```python
from build123d import *

# Parameters (mm, degrees)
F0_W     = 58
F0_H     = 36
F0_R     = 1.25
F0_R_2   = 1.2
F1_DEPTH = 9
F0_R_3   = 1
F2_DEPTH = 5.5
F3_DEPTH = 9
F4_R     = 3
F5_SIZE  = 2
F6_DEPTH = 10


with BuildPart() as f1:
    # F0 (on Top) → F1 (new body)
    with BuildSketch(Plane.XY):
        with Locations((22.1260370687, 12.181818096)):
            Rectangle(F0_W, F0_H)
        with Locations((-2.8739629313, -1.818181904)):
            Circle(F0_R, mode=Mode.SUBTRACT)
        with Locations((3.1260370687, -2.818181904)):
            Circle(F0_R_2, mode=Mode.SUBTRACT)
        with Locations((41.1260370687, -2.818181904)):
            Circle(F0_R_2, mode=Mode.SUBTRACT)
        with Locations((47.1260370687, -1.818181904)):
            Circle(F0_R, mode=Mode.SUBTRACT)
        with BuildLine():
            Line((-0.0042433119, 0.0237876128), (-0.0123524841, 0.02397218))
            Line((-0.0123524841, 0.02397218), (-0.0123524841, 0.0693824727))
            ThreePointArc((-0.0123524841, 0.0693824727), (-1.0671188126, 12.0466773263), (-0.0123524841, 24.02397218))
            ThreePointArc((-0.0123524841, 24.02397218), (22.4498159336, 26.0118318189), (44.9770614896, 25))
            ThreePointArc((44.9770614896, 25), (46.474513746, 12), (44.9770614896, -1))
            ThreePointArc((44.9770614896, -1), (22.4574664967, -1.8971785964), (0, 0))
            ThreePointArc((0, 0), (-0.0021227043, 0.0118936194), (-0.0042433119, 0.0237876128))
        make_face(mode=Mode.SUBTRACT)
        with Locations((-2.8739629313, 26.181818096)):
            Circle(F0_R, mode=Mode.SUBTRACT)
        with Locations((3.1260370687, 27.381818096)):
            Circle(F0_R_2, mode=Mode.SUBTRACT)
        with Locations((41.1260370687, 27.381818096)):
            Circle(F0_R_2, mode=Mode.SUBTRACT)
        with Locations((47.1260370687, 26.181818096)):
            Circle(F0_R, mode=Mode.SUBTRACT)
    extrude(amount=F1_DEPTH)

    # F0 (on Top) → F2 (join)
    with BuildSketch(Plane.XY):
        with BuildLine():
            Line((-0.0123524841, 24.02397218), (-0.0123524841, 0.0693824727))
            ThreePointArc((-0.0123524841, 0.0693824727), (-0.0083017494, 0.0465843578), (-0.0042433119, 0.0237876128))
            Line((-0.0042433119, 0.0237876128), (44.9770614896, -1))
            Line((44.9770614896, -1), (44.9770614896, 25))
            Line((44.9770614896, 25), (-0.0123524841, 24.02397218))
        make_face()
        with Locations((2.9444331303, 2.0848012064)):
            Circle(F0_R_3, mode=Mode.SUBTRACT)
        with Locations((41.6948273778, 2.0848012064)):
            Circle(F0_R_3, mode=Mode.SUBTRACT)
        with Locations((18.8074270263, 12.2937392443)):
            Circle(F0_R_3, mode=Mode.SUBTRACT)
        with Locations((2.9444331303, 21.6664075851)):
            Circle(F0_R_3, mode=Mode.SUBTRACT)
        with Locations((26.8074270263, 12.2937392443)):
            Circle(F0_R_3, mode=Mode.SUBTRACT)
        with Locations((41.6948273778, 21.6664075851)):
            Circle(F0_R_3, mode=Mode.SUBTRACT)
        with Locations((2.9444331303, 21.6664075851)):
            Circle(F0_R_3)
        with Locations((2.9444331303, 2.0848012064)):
            Circle(F0_R_3)
        with Locations((41.6948273778, 2.0848012064)):
            Circle(F0_R_3)
        with Locations((41.6948273778, 21.6664075851)):
            Circle(F0_R_3)
        with BuildLine():
            ThreePointArc((44.9770614896, 25), (22.4498159336, 26.0118318189), (-0.0123524841, 24.02397218))
            Line((-0.0123524841, 24.02397218), (44.9770614896, 25))
        make_face()
        with BuildLine():
            Line((44.9770614896, -1), (-0.0042433119, 0.0237876128))
            ThreePointArc((-0.0042433119, 0.0237876128), (-0.0021227043, 0.0118936194), (0, 0))
            ThreePointArc((0, 0), (22.4574664967, -1.8971785964), (44.9770614896, -1))
        make_face()
        with BuildLine():
            Line((44.9770614896, 25), (44.9770614896, -1))
            ThreePointArc((44.9770614896, -1), (46.474513746, 12), (44.9770614896, 25))
        make_face()
        with BuildLine():
            ThreePointArc((-0.0123524841, 24.02397218), (-1.0671188126, 12.0466773263), (-0.0123524841, 0.0693824727))
            Line((-0.0123524841, 0.0693824727), (-0.0123524841, 24.02397218))
        make_face()
    extrude(amount=F2_DEPTH)

    # F0 (on Top) → F3 (join)
    with BuildSketch(Plane.XY):
        with Locations((41.6948273778, 21.6664075851)):
            Circle(F0_R_3)
        with Locations((2.9444331303, 21.6664075851)):
            Circle(F0_R_3)
        with Locations((2.9444331303, 2.0848012064)):
            Circle(F0_R_3)
        with Locations((41.6948273778, 2.0848012064)):
            Circle(F0_R_3)
    extrude(amount=F3_DEPTH)

    # F4
    f4_edges = [f1.edges().sort_by_distance(p)[0] for p in [
        (51.126037, 30.181818, 4.5),
        (51.126037, -5.818182, 4.5),
        (-6.873963, -5.818182, 4.5),
        (-6.873963, 30.181818, 4.5),
    ]]
    fillet(f4_edges, radius=F4_R)

    # F5
    f5_edges = [f1.edges().sort_by_distance(p)[0] for p in [
        (-4.123963, -1.818182, 0),
        (-4.123963, 26.181818, 0),
        (45.876037, -1.818182, 0),
        (45.876037, 26.181818, 0),
    ]]
    chamfer(f5_edges, length=F5_SIZE)

    # F0 (on Top) → F6 (join)
    with BuildSketch(Plane.XY):
        with Locations((3.1260370687, 27.381818096)):
            Circle(F0_R_2)
        with Locations((3.1260370687, -2.818181904)):
            Circle(F0_R_2)
        with Locations((41.1260370687, -2.818181904)):
            Circle(F0_R_2)
        with Locations((41.1260370687, 27.381818096)):
            Circle(F0_R_2)
    extrude(amount=F6_DEPTH)


solid = f1.part
```
Read the model definition and answer for the solid it produces. Units are mm, in the model's axes. A direction names the side the tool comes from. Coordinates: 2 decimals unless noted, no trailing zeros. Loops run counter-clockwise (first coordinate to the right, second up) from the corner with the lowest first, then second, coordinate; pieces in that order, holes last. Notation, with made-up numbers: (19.25, 67) -> (56.25, 67) arc R13 ccw to (56.25, 83) -> close; hole circle Ø1 at (24.5, 29.5). An arc over 180 degrees is marked (long way). Return JSON: item names as keys, results as strings.
Item 1: Find section A-A (z = 6.5). Count the separate pieces of the cut face and the enclosed holes in it, plus the area to 3 significant figures.
Answers:
{"separate pieces": "5", "enclosed holes": "5", "area": "818 mm2"}
Item 2: For faces 5 (the cylindrical face through (-3.14, 24.96, 5.45)), 6 (the flat face through (42, 22, 9)), 7 (the cylindrical face through (42.235, -3.278, 9.493)), determine the directions among +Z, -Z, +X, -X, +Y, -Y from which every point of the face is accessible in a straight line to the end or side of a thin tool.
Answers:
{"face 5": "+Z, -Z", "face 6": "+Z, +X, -X", "face 7": "+Z"}
Item 3: Find the intervals of material crossed by probe 1 along X at (y, z) = (26, 2.5); probe 2 along X at (y, z) = (-1, 3.5); probe 3 along Z at (x, y) = (0.5, 13.5), in increasing order.
Answers:
{"probe 1": "x = -6.87 to -4.11, -1.64 to 45.89, 48.36 to 51.13", "probe 2": "x = -6.87 to -3.82, -1.93 to 46.18, 48.07 to 51.13", "probe 3": "z = 0 to 5.5"}
Item 4: Flat-ended cylindrical pins translate along their axes: P1, Ø8.5, axis at x = 27.5, y = 16, coming from the +Z side; P2, Ø3, axis at x = 47.13, y = -1.82, coming from the -Z side; P3, Ø1, axis at x = 24, y = 17.5, coming from the -Z side; P4, Ø1, axis at x = 17.5, y = 26, coming from the +Z side. Find the tip coordinate at first contact, or state that the pin passes through.
Answers:
{"P1": "stops at z = 5.5", "P2": "stops at z = 1.75", "P3": "stops at z = 0", "P4": "stops at z = 9"}
Item 5: For a pull along X with two mould halves and no side action, classify faces 1 (the flat face through (51.126, 12, 4)), 2 (the flat face through (41, 27, 10)), 3 (the cylindrical face through (4.27, -2.46, 9.49)), 4 (the cylindrical face through (-6.018, -4.916, 4.563)) as +X half, -X half, draft (parallel to the pull), parting line (faces both ways), or undercut.
Answers:
{"face 1": "+X half", "face 2": "draft", "face 3": "undercut", "face 4": "-X half"}
Item 6: Find section D-D (y = 16). Determine the outline of the cut face in (x, z).
Answers:
{"outline": "(-6.87, 0) -> (51.13, 0) -> (51.13, 9) -> (46.33, 9) -> (46.33, 5.5) -> (-0.95, 5.5) -> (-0.95, 9) -> (-6.87, 9) -> close"}
Item 7: Find section B-B (x = 3). Determine the outline of the cut face in (y, z).
Answers:
{"outline": "(-5.82, 0) -> (30.18, 0) -> (30.18, 9) -> (28.58, 9) -> (28.58, 10) -> (26.19, 10) -> (26.19, 9) -> (24.47, 9) -> (24.47, 5.5) -> (22.66, 5.5) -> (22.66, 9) -> (20.67, 9) -> (20.67, 5.5) -> (3.08, 5.5) -> (3.08, 9) -> (1.09, 9) -> (1.09, 5.5) -> (-0.42, 5.5) -> (-0.42, 9) -> (-1.62, 9) -> (-1.62, 10) -> (-4.01, 10) -> (-4.01, 9) -> (-5.82, 9) -> close"}
